Job drawing, mm, ordinate dimensions from the low corner. One solid piece. Coordinates: 2 decimals unless noted, no trailing zeros. Write each loop counter-clockwise with the first axis right and the second up, starting at its lowest first coordinate (ties: lowest second). Pieces come first, ordered by that corner, then holes.
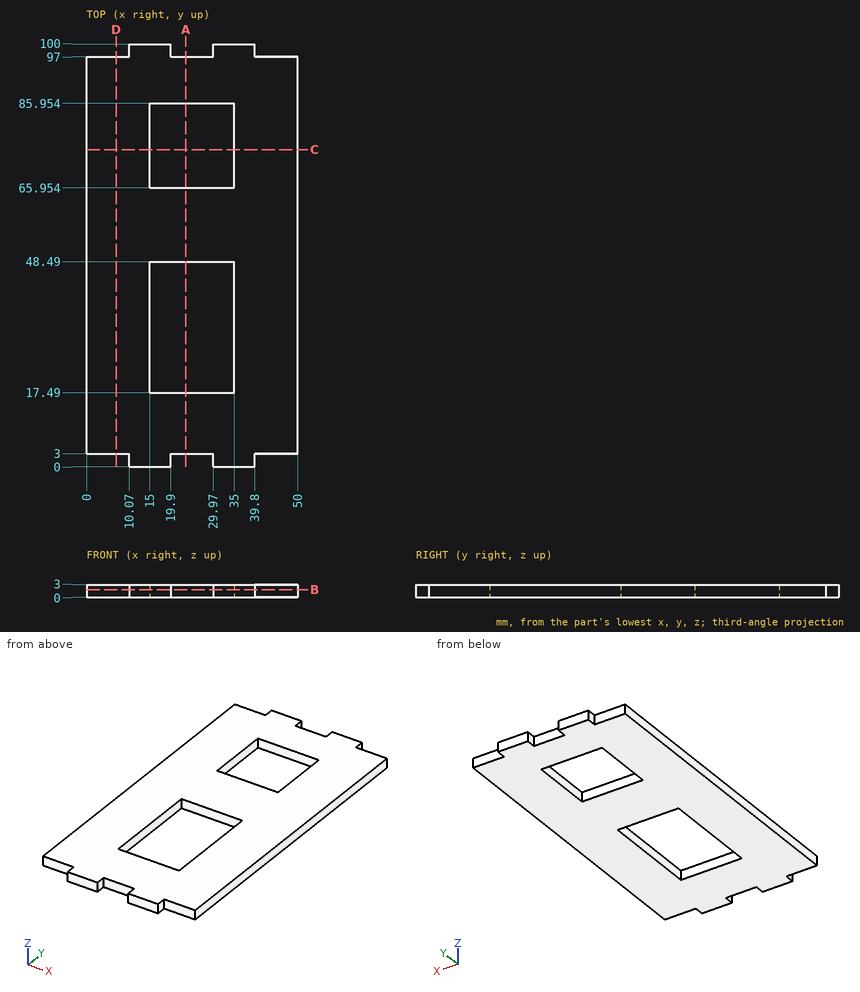
1. Probe line 1 along Y through (x, z) = (32, 0.3); line 2 along X through (y, z) = (79, 0.95); line 3 along Y through (x, z) = (24.5, 2.75). List the from-to ranges inside material, lowest first.
Computed values:
line 1: y = 0 to 17.49, 48.49 to 65.95, 85.95 to 100
line 2: x = 0 to 15, 35 to 50
line 3: y = 3 to 17.49, 48.49 to 65.95, 85.95 to 97
2. Flat gauge pins, fed straight in: pin 1 (1.5 mm diameter, centred on x = 46, z = 1.5, fed in from +Y); pin 2 (1.5 mm diameter, centred on y = 98.5, z = 1.5, fed in from -X). Where does each tip first touch, or does it go through?
Computed values:
pin 1: stops at y = 97
pin 2: stops at x = 10.07
3. Saw through at C-C on y = 75. List the corners of the cut face in (x, z), plus the area to 3 significant figures.
Computed values:
outline: (0, 0) - (15, 0) - (15, 3) - (0, 3) - close; (35, 0) - (50, 0) - (50, 3) - (35, 3) - close
area: 90.0 mm2
4. Saw through at B-B on z = 1.8. List the corners of the cut face in (x, y).
Computed values:
outline: (0, 3) - (10.07, 3) - (10.07, 0) - (19.9, 0) - (19.9, 3) - (29.97, 3) - (29.97, 0) - (39.8, 0) - (39.8, 3) - (50, 3) - (50, 97) - (39.8, 97) - (39.8, 100) - (29.97, 100) - (29.97, 97) - (19.9, 97) - (19.9, 100) - (10.07, 100) - (10.07, 97) - (0, 97) - close; hole (15, 17.49) - (35, 17.49) - (35, 48.49) - (15, 48.49) - close; hole (15, 65.95) - (35, 65.95) - (35, 85.95) - (15, 85.95) - close
5. Saw through at D-D on x = 7. List the corners of the cut face in (y, z).
Computed values:
outline: (3, 0) - (97, 0) - (97, 3) - (3, 3) - close
6. Saw through at A-A on x = 23.5. List the corners of the cut face in (y, z), plus the area to 3 significant figures.
Computed values:
outline: (3, 0) - (17.49, 0) - (17.49, 3) - (3, 3) - close; (48.49, 0) - (65.95, 0) - (65.95, 3) - (48.49, 3) - close; (85.95, 0) - (97, 0) - (97, 3) - (85.95, 3) - close
area: 129 mm2
